```python
from build123d import *

# Parameters (mm, degrees)
BOSS_EXTRUDE1_DEPTH = 22.225
SKETCH2_R           = 2.5
SKETCH2_R_2         = 7.5
CUT_EXTRUDE5_DEPTH  = 18
CUT_EXTRUDE7_START  = 12
SKETCH2_8_R         = 15.5
CUT_EXTRUDE7_DEPTH  = 42


with BuildPart() as part:
    # Sketch1 → Boss-Extrude1 (new body, symmetric)
    with BuildSketch(Plane.XY):
        with BuildLine():
            Line((0, 28), (0, -122))
            ThreePointArc((0, -122), (3.91238571, -129.933533403), (12.588190451, -131.659258263))
            Line((12.588190451, -131.659258263), (49.294095226, -121.823940721))
            ThreePointArc((49.294095226, -121.823940721), (52.263200822, -119.606804413), (52.890738004, -115.954753136))
            Line((52.890738004, -115.954753136), (51.18308621, -107.920883092))
            ThreePointArc((51.18308621, -107.920883092), (47.694814113, -102.228540385), (41.401610203, -100))
            Line((41.401610203, -100), (23, -100))
            ThreePointArc((23, -100), (19.464466094, -98.535533906), (18, -95))
            Line((18, -95), (18, 12))
            ThreePointArc((18, 12), (18.585786438, 13.414213562), (20, 14))
            Line((20, 14), (21, 14))
            ThreePointArc((21, 14), (22.414213562, 14.585786438), (23, 16))
            Line((23, 16), (23, 28))
            Line((23, 28), (18, 28))
            Line((18, 28), (0, 28))
        make_face()
        with BuildLine():
            Line((4, -111), (4, -90))
            ThreePointArc((4, -90), (9, -85), (14, -90))
            Line((14, -90), (14, -111))
            ThreePointArc((14, -111), (9, -116), (4, -111))
        make_face(mode=Mode.SUBTRACT)
        with BuildLine():
            Line((4, -69), (4, -39))
            ThreePointArc((4, -39), (9, -34), (14, -39))
            Line((14, -39), (14, -69))
            ThreePointArc((14, -69), (9, -74), (4, -69))
        make_face(mode=Mode.SUBTRACT)
        with BuildLine():
            Line((29.708099244, -108.5), (36.291900756, -108.5))
            ThreePointArc((36.291900756, -108.5), (44, -110), (36.291900756, -111.5))
            Line((36.291900756, -111.5), (29.708099244, -111.5))
            ThreePointArc((29.708099244, -111.5), (22, -110), (29.708099244, -108.5))
        make_face(mode=Mode.SUBTRACT)
        Polygon((4, 12), (4, -12), (12, -14), (12, 14), align=None, mode=Mode.SUBTRACT)
    extrude(amount=BOSS_EXTRUDE1_DEPTH, both=True)

    # Sketch2 → Cut-Extrude5 (cut)
    with BuildSketch(Plane(origin=(0, 0, 0), x_dir=(0, 0, -1), z_dir=(1, 0, 0))):
        with Locations((14, -78)):
            Circle(SKETCH2_R)
        with Locations((-14, -78)):
            Circle(SKETCH2_R)
        with Locations((-14, -25)):
            Circle(SKETCH2_R)
        with Locations((14, -25)):
            Circle(SKETCH2_R)
        Circle(SKETCH2_R_2)
    extrude(amount=CUT_EXTRUDE5_DEPTH, mode=Mode.SUBTRACT)

    # Sketch2<8> → Cut-Extrude7 (cut, through all)
    with BuildSketch(Plane(origin=(0, 0, 0), x_dir=(0, 0, -1), z_dir=(1, 0, 0)).offset(CUT_EXTRUDE7_START)):
        Circle(SKETCH2_8_R)
    extrude(amount=CUT_EXTRUDE7_DEPTH, mode=Mode.SUBTRACT)


solid = part.part
```
CAD build for the part. Positions are in the model's coordinates, mm. A direction names the side the tool comes from. Give positions to 0.01 mm unless a question says otherwise; leave off trailing zeros. Loops run counter-clockwise (first coordinate to the right, second up) from the corner with the lowest first, then second, coordinate; pieces in that order, holes last. Notation, with made-up numbers: (49, -19.75) - (95, -19.75) arc R24 ccw to (95, 0.25) - close; hole circle Ø11 at (83.5, 86.25). An arc over 180 degrees is marked (long way). Put each result on its own line as item: value.
Q1. Probe line 1 along X through (y, z) = (-59, 9.5); line 2 along Y through (x, z) = (9.5, -20) (1 decimal); line 3 along X through (y, z) = (9.5, -15.5). List the from-to ranges inside material, lowest first.
Filled in:
line 1: x = 0 to 4, 14 to 18
line 2: y = -132 to -116, -85 to -74, -34 to -13.4, 13.4 to 28
line 3: x = 0 to 4, 12 to 18
Q2. Slice it at D-D (x = 26). Give the cut face in (y, z) (3 decimals), plus the area to 3 significant figures.
Filled in:
outline: (-128.066, -22.225) - (-114, -22.225) - (-114, 22.225) - (-128.066, 22.225) - close; (-106, -22.225) - (-100, -22.225) - (-100, 22.225) - (-106, 22.225) - close
area: 892 mm²
Q3. Slice it at A-A (y = -78). Give the cut face in (x, z) (3 decimals), plus the area to 3 significant figures.
Filled in:
outline: (0, -22.225) - (18, -22.225) - (18, -16.5) - (0, -16.5) - close; (0, -11.5) - (18, -11.5) - (18, 11.5) - (0, 11.5) - close; (0, 16.5) - (18, 16.5) - (18, 22.225) - (0, 22.225) - close
area: 620 mm²
Q4. Slice it at B-B (z = 14). Give the number of separate pieces and of enclosed holes in the cut face, plus the area to 3 significant figures.
Filled in:
separate pieces: 3
enclosed holes: 3
area: 2,520 mm²
Q5. Tool access for faces 1 (the face through (9, -85, 0)), 2 (the face through (18, -42, 0)), 3 (the face through (1.972, 0.33, 7.493)): list every direction of +Z, -Z, +X, -X, +Y, -Y with a clear straight run to the whole face (end or side of a thin tool).
Filled in:
face 1: +Z, -Z
face 2: +Z, -Z, +X
face 3: +X, -X
Q6. Flat gauge pins, fed straight in: pin 1 (1 mm diameter, centred on x = 28.5, z = -11.5, fed in from +Y); pin 2 (2 mm diameter, centred on y = -3, z = 9, fed in from -X); pin 3 (1.7 mm diameter, centred on y = 15, z = 0, fed in from +X); pin 4 (1.5 mm diameter, centred on x = 44, y = -98.5, fed in from +Z). Where does each tip first touch, or does it go through?
Filled in:
pin 1: stops at y = -100
pin 2: stops at x = 0
pin 3: stops at x = 22.99
pin 4: passes through
Q7. Mould opens along Y. For faces 4 (the face through (14.4, -68.7, 22.225)), 5 (the face through (9, -34, 0)), 6 (the face through (47.77, -102.29, 0.31)) say: pulls with the +Y half, pulls with the -Y half, needs draft (parallel to the pull), parting line crosses it, or undercut.
Filled in:
face 4: needs draft
face 5: undercut
face 6: pulls with the +Y half
